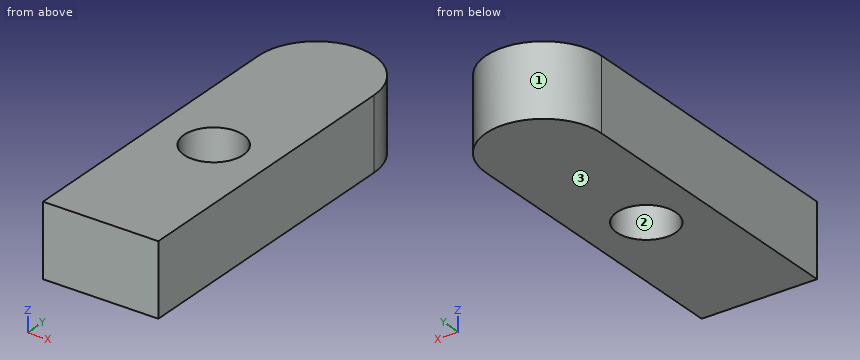
```python
from build123d import *

# Parameters (mm, degrees)
SKETCH_1_R      = 2.05
EXTRUDE_1_DEPTH = 2.5


with BuildPart() as part:
    # 스케치1 → 보스-돌출1 (new, symmetric)
    with BuildSketch(Plane.XY):
        with BuildLine():
            Line((-4, 0), (-4, 10))
            ThreePointArc((-4, 10), (0, 14), (4, 10))
            Line((4, 10), (4, 0))
            Line((4, 0), (4, -11.014558485))
            Line((4, -11.014558485), (-4, -11.014558485))
            Line((-4, -11.014558485), (-4, 0))
        make_face()
        Circle(SKETCH_1_R, mode=Mode.SUBTRACT)
    extrude(amount=EXTRUDE_1_DEPTH, both=True)


solid = part.part
```
Check sheet for the modelled part. Datum: model origin and axes. Units: mm. Face numbers are marked on the shaded views. Coordinates: 2 decimals unless noted, no trailing zeros. Order: outer loops, then holes, each group sorted by start corner. A loop starts at its lowest first (then second) coordinate and runs counter-clockwise, first axis right, second up. Notation, with made-up numbers: (-13, 51) -> (0, 51) arc R7 cw to (0, 62) -> close; hole circle Ø11 at (-28, 34). An arc over 180 degrees is marked (long way). Write item = value, one per line. Start each with the question number.
1) Cross-section at D-D (x = 2.5). Enter the section's corners in (y, z).
2) Cross-section at B-B (y = 0). Enter the section's corners in (x, z).
3) Cross-section at C-C (z = -1.55). Enter the section's corners in (x, y), then the cut area to 3 significant figures.
4) Cross-section at A-A (x = 0). Enter the section's corners in (y, z), then the cut area to 3 significant figures.
5) Go/stop test with flat-tipped pins: P1, Ø2.5, axis at x = 0, y = 0, coming from the +Z side; P2, Ø1.5, axis at x = -3, z = 1.5, coming from the +Y side. Record where each tip stops, or that it passes through.
6) Mould release check, pull along Y, two halves, no side actions. Record for the marked faces 1, 2 and 3: +Y half, -Y half, draft (parallel to the pull), parting line (faces both ways), or undercut.
7) Material ranges on L1, parallel to Y at x = 0, z = -0.05; L2, parallel to Y at x = -2.5, z = 1.7; L3, parallel to Y at x = -1.5, z = -1.6, recorded low to high.
Ans:
q1.outline = (-11.01, -2.5) -> (13.12, -2.5) -> (13.12, 2.5) -> (-11.01, 2.5) -> close
q2.outline = (-4, -2.5) -> (-2.05, -2.5) -> (-2.05, 2.5) -> (-4, 2.5) -> close; (2.05, -2.5) -> (4, -2.5) -> (4, 2.5) -> (2.05, 2.5) -> close
q3.outline = (-4, -11.01) -> (4, -11.01) -> (4, 10) arc R4 ccw to (-4, 10) -> close; hole circle Ø4.1 at (0, 0)
q3.area = 180 mm²
q4.outline = (-11.01, -2.5) -> (-2.05, -2.5) -> (-2.05, 2.5) -> (-11.01, 2.5) -> close; (2.05, -2.5) -> (14, -2.5) -> (14, 2.5) -> (2.05, 2.5) -> close
q4.area = 105 mm²
q5.P1 = through
q5.P2 = 13.31
q6.face_1 = +Y half
q6.face_2 = undercut
q6.face_3 = draft
q7.L1 = -11.01 to -2.05, 2.05 to 14
q7.L2 = -11.01 to 13.12
q7.L3 = -11.01 to -1.4, 1.4 to 13.71
